For this review, take the finished solid that the model builds, in its own axes (mm). Coordinates: 2 decimals unless noted, no trailing zeros. Loops run counter-clockwise (first coordinate to the right, second up) from the corner with the lowest first, then second, coordinate; pieces in that order, holes last. Notation, with made-up numbers: (80, 47.5) -> (115, 47.5) arc R12 cw to (115, 69.5) -> close; hole circle Ø4 at (-9.5, 31). An arc over 180 degrees is marked (long way). One line per item, written item: value.
from build123d import *

# Parameters (mm, degrees)
BOSS_EXTRUDE1_DEPTH   = 1.5875
F_2_CLEARANCE_HOLE1_D = 2.7051
CUT_EXTRUDE1_DEPTH    = 2.5875


with BuildPart() as part:
    # Sketch1 → Boss-Extrude1 (new body)
    with BuildSketch(Plane.XY):
        with BuildLine():
            Line((-52.648603939, -67.272400153), (-30.578425, -43.620868829))
            Line((-30.578425, -43.620868829), (-18.837275, -31.03845263))
            Line((-18.837275, -31.03845263), (-18.837275, 15.096748243))
            Line((-18.837275, 15.096748243), (-18.837275, 22.917825485))
            Line((-18.837275, 22.917825485), (-5.036497092, 22.917825485))
            ThreePointArc((-5.036497092, 22.917825485), (16.456769026, -18.908795935), (23.866475, -65.347174515))
            Line((23.866475, -65.347174515), (23.866475, -73.221174515))
            Line((23.866475, -73.221174515), (-30.578425, -73.221174515))
            Line((-30.578425, -73.221174515), (-52.355372399, -73.221174515))
            ThreePointArc((-52.355372399, -73.221174515), (-54.684874047, -71.693608254), (-54.212432291, -68.948278512))
            Line((-54.212432291, -68.948278512), (-52.648603939, -67.272400153))
        make_face()
    extrude(amount=BOSS_EXTRUDE1_DEPTH)

    # #2 Clearance Hole1 (through all)
    with Locations(Plane(origin=(0, 0, 0), x_dir=(-1, 0, 0), z_dir=(0, 0, -1))):
        with Locations((-21.834475, -71.189174515), (52.355372399, -70.681174515), (11.936886046, 20.885825485)):
            Hole(F_2_CLEARANCE_HOLE1_D / 2)

    # Sketch4 → Cut-Extrude1 (cut, through all)
    with BuildSketch(Plane(origin=(0, 0, 0), x_dir=(-1, 0, 0), z_dir=(0, 0, -1))):
        with BuildLine():
            ThreePointArc((-21.881749979, -41.090174515), (-23.369466076, -53.178144332), (-23.866475, -65.347174515))
            Line((-23.866475, -65.347174515), (-14.277975, -65.347174515))
            Line((-14.277975, -65.347174515), (-14.277975, -41.090174515))
            Line((-14.277975, -41.090174515), (-21.881749979, -41.090174515))
        make_face()
        with BuildLine():
            ThreePointArc((-5.845175, 5.742133621), (-15.818945129, -17.004413391), (-21.881749979, -41.090174515))
            Line((-21.881749979, -41.090174515), (-14.277975, -41.090174515))
            Line((-14.277975, -41.090174515), (-5.845175, -41.090174515))
            Line((-5.845175, -41.090174515), (-5.845175, 5.742133621))
        make_face()
        with BuildLine():
            ThreePointArc((5.036497092, 22.917825485), (-0.665836205, 14.565033613), (-5.789292349, 5.845175))
            Line((-5.789292349, 5.845175), (5.036497092, 5.845175))
            Line((5.036497092, 5.845175), (5.036497092, 22.917825485))
        make_face()
    extrude(amount=-CUT_EXTRUDE1_DEPTH, mode=Mode.SUBTRACT)


solid = part.part
1. Take a section at B-B, the plane y = -29. Give the boundary of the cut face in (x, z), and give its area (3 significant figures).
Return value:
outline: (-18.84, 0) -> (5.85, 0) -> (5.85, 1.59) -> (-18.84, 1.59) -> close
area: 39.2 mm2
2. Take a section at A-A, the plane z = 0.6. Give the number of separate pieces and of enclosed holes in the cut face, and give its area (3 significant figures).
Return value:
separate pieces: 1
enclosed holes: 3
area: 3,340 mm2
3. The part is to be moulded in two halves that separate along Y. For faces 1 (the cylindrical face through (-54.67, -71.73, 0.78)), 2 (the flat face through (-15, -35, 0)), 3 (the cylindrical face through (-52.65, -72, 0.8)), say which applies: pulls with the +Y half, pulls with the -Y half, needs draft (parallel to the pull), parting line crosses it, or undercut.
Return value:
face 1: parting line crosses it
face 2: needs draft
face 3: undercut
4. Insertion check: pin 1 Ø0.5 at (y, z) = (13, 1) entering from +X; pin 2 Ø1 at (x, y) = (4.5, -24) entering from -Z; pin 3 Ø0.8 at (x, z) = (0, 1) entering from +Y. Each pin has a flat end and moves straight along its axis. Give the tip position at first contact, or say it passes through.
Return value:
pin 1: stops at x = -5.04
pin 2: stops at z = 0
pin 3: stops at y = 5.85
5. To check wall thickness, follow probe 1 along X at (y, z) = (9.5, 1.15); probe 2 along Y at (x, z) = (-2.5, 0.7); probe 3 along X at (y, z) = (-19, 1.5). State the ranges of each line that lie inside material, in increasing order. Write a range as from..to.
Return value:
probe 1: x = -18.84..-5.04
probe 2: y = -73.22..5.85
probe 3: x = -18.84..5.85
6. Take a section at C-C, the plane x = 9.5. Give the boundary of the cut face in (y, z), and give its area (3 significant figures).
Return value:
outline: (-73.22, 0) -> (-41.09, 0) -> (-41.09, 1.59) -> (-73.22, 1.59) -> close
area: 51.0 mm2
